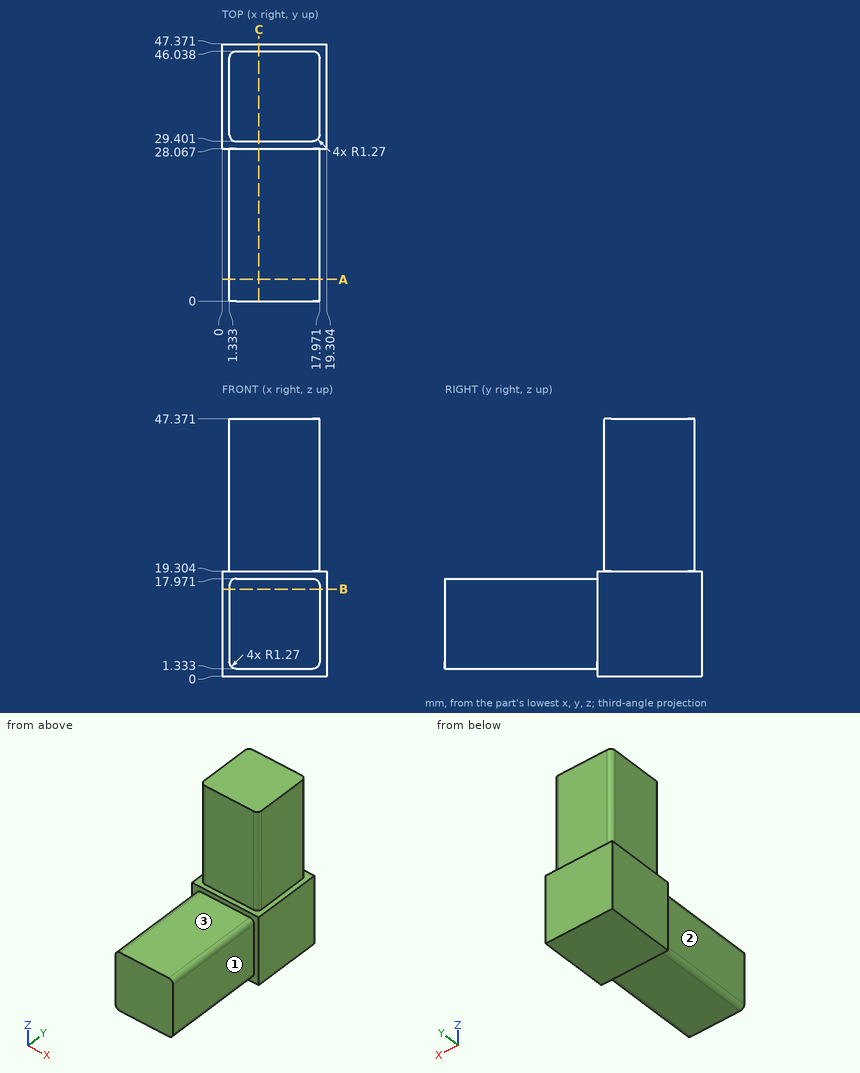
Verification items for this drawing (mm, ordinates from the low corner). A direction names the side the tool comes from. Coordinates: 2 decimals unless noted, no trailing zeros. Write each loop counter-clockwise with the first axis right and the second up, starting at its lowest first coordinate (ties: lowest second). Pieces come first, ordered by that corner, then holes. Notation, with made-up numbers: M -34,-9 L -12,-9 A8 ccw -12,-4 Z; hole C 65,23 d10. An arc over 180 degrees is marked long. Use one line per item in the form item = value. Start each with the question number.
1) Thickness scan on probe 1 along Z at (x, y) = (4.75, 17); probe 2 along Y at (x, z) = (4.25, 32). Record the ranges inside material, lowest first. Write a range as from..to.
2) Section check C-C on x = 6.75. Enter the section's corners in (y, z) (1 decimal), and give its area (3 significant figures).
3) Go/stop test with flat-tipped pins: pin 1 Ø2 at (x, y) = (15.5, 27) entering from +Z; pin 2 Ø4 at (y, z) = (36, 31) entering from +X; pin 3 Ø7 at (x, z) = (10.5, 37.5) entering from -Y. Record where each tip stops, or that it passes through.
4) Section check B-B on z = 16. Enter the section's corners in (x, y) (1 decimal).
5) Section check A-A on y = 4. Enter the section's corners in (x, z).
6) Set-up check for the marked faces 1, 2 and 3: record each of +Z, -Z, +X, -X, +Y, -Y from which the full face is reachable in a straight line by a thin tool's end or side.
Responses:
q1.probe_1 = 1.33..17.97
q1.probe_2 = 29.4..46.04
q2.outline = M 0,1.3 L 28.1,1.3 L 28.1,0 L 47.4,0 L 47.4,19.3 L 46,19.3 L 46,47.4 L 29.4,47.4 L 29.4,19.3 L 28.1,19.3 L 28.1,18 L 0,18 Z
q2.area = 1,310 mm2
q3.pin_1 = 17.97
q3.pin_2 = 17.97
q3.pin_3 = 29.4
q4.outline = M 0,28.1 L 1.3,28.1 L 1.3,0 L 18,0 L 18,28.1 L 19.3,28.1 L 19.3,47.4 L 0,47.4 Z
q5.outline = M 1.33,2.6 A1.27 ccw 2.6,1.33 L 16.7,1.33 A1.27 ccw 17.97,2.6 L 17.97,16.7 A1.27 ccw 16.7,17.97 L 2.6,17.97 A1.27 ccw 1.33,16.7 Z
q6.face_1 = +Z, -Z, +X, -Y
q6.face_2 = +Z, -Z, -X, -Y
q6.face_3 = +Z, +X, -X, -Y
